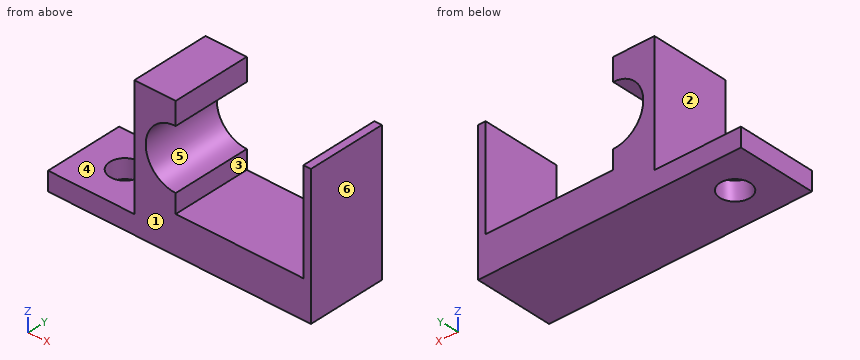
from build123d import *

# Parameters (mm, degrees)
F0_W     = 70
F0_H     = 21
F1_DEPTH = 37
F2_W     = 34
F2_H     = 21
F3_DEPTH = 27
F5_DEPTH = 21
F6_W     = 23
F6_H     = 21
F7_DEPTH = 32
F9_D     = 8


with BuildPart() as f1:
    # F0 (on Top) → F1 (new body)
    with BuildSketch(Plane.XY):
        with Locations((-50.1195863448, 2.1268057005)):
            Rectangle(F0_W, F0_H)
    extrude(amount=F1_DEPTH)

    # F2 (on face) → F3 (cut)
    with BuildSketch(Plane.XY.offset(37)):
        with Locations((-34.1195863448, 2.1268057005)):
            Rectangle(F2_W, F2_H)
    extrude(amount=-F3_DEPTH, mode=Mode.SUBTRACT)

    # F4 (on face) → F5 (cut)
    with BuildSketch(Plane.XZ.offset(8.3731942995)):
        with BuildLine():
            Line((-51.1195863448, 15), (-51.1195863448, 31))
            ThreePointArc((-51.1195863448, 31), (-59.1195863448, 23), (-51.1195863448, 15))
        make_face()
    extrude(amount=-F5_DEPTH, mode=Mode.SUBTRACT)

    # F6 (on face) → F7 (cut)
    with BuildSketch(Plane.XY.offset(37)):
        with Locations((-73.6195863448, 2.1268057005)):
            Rectangle(F6_W, F6_H)
    extrude(amount=-F7_DEPTH, mode=Mode.SUBTRACT)

    # F9 (through all)
    with Locations(Plane.XY.offset(5)):
        with Locations((-74.1195863448, 2.1268057005)):
            Hole(F9_D / 2)


solid = f1.part
Input: part model. Units: mm. Frame: model coordinates. Face numbers are marked on the shaded views. A direction names the side the tool comes from. Give positions to 0.01 mm unless a question says otherwise; leave off trailing zeros. Order: outer loops, then holes, each group sorted by start corner. A loop starts at its lowest first (then second) coordinate and runs counter-clockwise, first axis right, second up.
Q1. Contact query for flat-ended pins moving along their axis: pin 1 Ø6.5 at (x, y) = (-31.5, 6) entering from +Z; pin 2 Ø6.5 at (x, y) = (-79, -3) entering from +Z; pin 3 Ø3 at (y, z) = (-0.5, 31) entering from -X. Output: stop coordinate, or through.
Checked values:
pin 1: stops at z = 10
pin 2: stops at z = 5
pin 3: stops at x = -62.12
Q2. Section C-C on x = -53. Output: boundary loops of the cut face in (y, z).
Checked values:
outline: (-8.37, 0) - (12.63, 0) - (12.63, 15.22) - (-8.37, 15.22) - close; (-8.37, 30.78) - (12.63, 30.78) - (12.63, 37) - (-8.37, 37) - close
Q3. Ray query, probe 1 along Z at (x, y) = (-26.5, 5); probe 2 along X at (y, z) = (8, 32.5); probe 3 along X at (y, z) = (7.75, 16). Return the intervals inside material, ascending.
Checked values:
probe 1: z = 0 to 10
probe 2: x = -62.12 to -51.12, -17.12 to -15.12
probe 3: x = -62.12 to -54.99, -17.12 to -15.12
Q4. Section B-B on y = -5. Output: boundary loops of the cut face in (x, z).
Checked values:
outline: (-85.12, 0) - (-15.12, 0) - (-15.12, 37) - (-17.12, 37) - (-17.12, 10) - (-51.12, 10) - (-51.12, 15) arc R8 cw to (-51.12, 31) - (-51.12, 37) - (-62.12, 37) - (-62.12, 5) - (-85.12, 5) - close
Q5. Section A-A on z = 23. Output: boundary loops of the cut face in (x, y).
Checked values:
outline: (-62.12, -8.37) - (-59.12, -8.37) - (-59.12, 12.63) - (-62.12, 12.63) - close; (-17.12, -8.37) - (-15.12, -8.37) - (-15.12, 12.63) - (-17.12, 12.63) - close
Q6. Draft query along X for the marked faces 4, 5 and 6. Return one class per face: +X half, -X half, draft (parallel to the pull), parting line (faces both ways), or undercut.
Checked values:
face 4: draft
face 5: undercut
face 6: +X half
Q7. Section D-D on y = -1. Output: boundary loops of the cut face in (x, z).
Checked values:
outline: (-85.12, 0) - (-76.61, 0) - (-76.61, 5) - (-85.12, 5) - close; (-71.62, 0) - (-15.12, 0) - (-15.12, 37) - (-17.12, 37) - (-17.12, 10) - (-51.12, 10) - (-51.12, 15) arc R8 cw to (-51.12, 31) - (-51.12, 37) - (-62.12, 37) - (-62.12, 5) - (-71.62, 5) - close
Q8. Set-up query: the marked faces 1, 2 and 3. Return all of +Z, -Z, +X, -X, +Y, -Y with unobstructed straight access to the full face (end or side cutting, diameter ignored); none if empty.
Checked values:
face 1: +Z, -Z, +X, -X, -Y
face 2: +Z, -X, +Y, -Y
face 3: +Z, +Y, -Y
